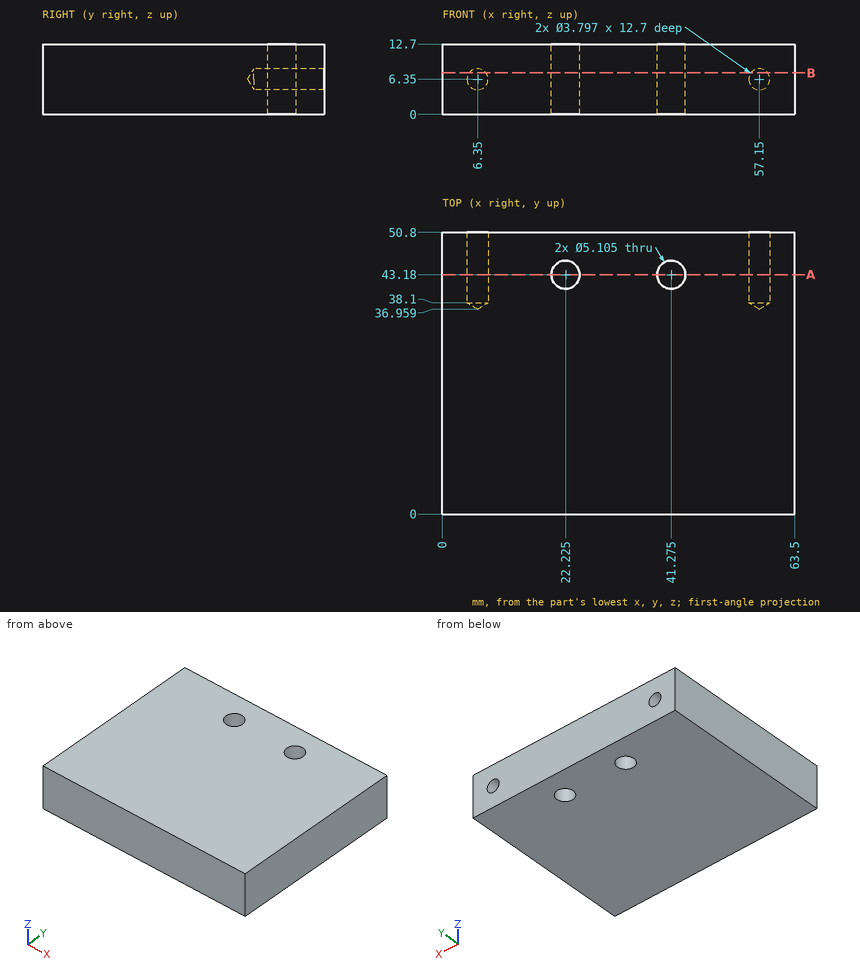
For this review, use the dimensioned drawing (mm, ordinates from the lowest corner) and the shaded views. Give positions to 0.01 mm unless a question says otherwise; leave off trailing zeros. Order: outer loops, then holes, each group sorted by start corner. A loop starts at its lowest first (then second) coordinate and runs counter-clockwise, first axis right, second up. Notation, with made-up numbers: M -6.75,48 L -0.75,48 A38 cw -0.75,87 Z; hole C -19.5,49.25 d6. An arc over 180 degrees is marked long. Use one line per item in the form item = value. Start each with the question number.
Item 1: To check wall thickness, follow line 1 along X through (y, z) = (44.5, 11.25); line 2 along Y through (x, z) = (21.5, 9.75); line 3 along Z through (x, y) = (6, 47) (1 decimal). State the ranges of each line that lie inside material, in increasing order. Write a range as from..to.
Item 2: We need section A-A on y = 43.18. Give the boundary of the cut face in (x, z).
Item 3: Insertion check: pin 1 Ø3 at (x, z) = (6.35, 6.35) entering from +Y. The pin has a flat end and moves straight along its axis. Give the tip position at first contact, or say it passes through.
Item 4: We need section B-B on z = 7.5. Give the number of separate pieces and of enclosed holes in the cut face, plus the area to 3 significant figures.
Completed:
q1.line_1 = 0..20.04, 24.41..39.09, 43.46..63.5
q1.line_2 = 0..40.73, 45.63..50.8
q1.line_3 = 0..4.5, 8.2..12.7
q2.outline = M 0,0 L 19.67,0 L 19.67,12.7 L 0,12.7 Z; M 24.78,0 L 38.72,0 L 38.72,12.7 L 24.78,12.7 Z; M 43.83,0 L 63.5,0 L 63.5,12.7 L 43.83,12.7 Z; hole C 6.35,6.35 d3.8; hole C 57.15,6.35 d3.8
q3.pin_1 = 37.86
q4.separate_pieces = 1
q4.enclosed_holes = 2
q4.area = 3,110 mm²
